Read the model definition and answer for the solid it produces. Units are mm, in the model's axes. A direction names the side the tool comes from. Coordinates: 2 decimals unless noted, no trailing zeros. Loops run counter-clockwise (first coordinate to the right, second up) from the corner with the lowest first, then second, coordinate; pieces in that order, holes last. Notation, with made-up numbers: M -0.75,75.25 L 18.25,75.25 A23 ccw 18.25,99.25 Z; hole C -33,81.25 d1. An arc over 180 degrees is marked long. One line per item, written item: value. Start each with the question number.
Autodesk Inventor part; units mm, degrees
ref_plane "YZ Plane" through (0, 0, 0) normal (1, 0, 0) x (0, 1, 0)
ref_plane "XZ Plane" through (0, 0, 0) normal (0, 1, 0) x (-1, 0, 0)
ref_plane "XY Plane" through (0, 0, 0) normal (0, 0, 1) x (1, 0, 0)
sketch "Sketch1" plane through (0, 0, 0) normal (0, 0, 1) x (1, 0, 0)
  line L0 (-20, 22.5) -> (20, 22.5)
  line L1 (20, 22.5) -> (20, -100)
  line L2 (20, -100) -> (-20, -100)
  line L3 (-20, -100) -> (-20, 22.5)
  circle A0 centre (0, 0) radius 4
  dimension "d0" = 122.5
  dimension "d1" = 40
  dimension "d2" = 20
  dimension "d3" = 22.5
  dimension "d4" = 8
extrude "Extrusion1" add sketch "Sketch1" along normal blind 5
sketch "Sketch2" plane through (0, 0, 5) normal (0, 0, 1) x (1, 0, 0)
  line L0 (20, 22.5) -> (-20, 22.5)
  line L1 (-20, -100) -> (20, -100)
  line L2 (-20, 22.5) -> (20, 22.5)
  line L3 (20, 22.5) -> (20, -100)
  line L4 (20, -100) -> (-20, -100)
  line L5 (-20, -100) -> (-20, 22.5)
  line L6 (-15, 17.5) -> (15, 17.5)
  line L7 (15, 17.5) -> (15, -95)
  line L8 (15, -95) -> (-15, -95)
  line L9 (-15, -95) -> (-15, 17.5)
  point P0 (0, 0)
  dimension "d7" = 5
  dimension "d8" = 5
  dimension "d9" = 5
  dimension "d10" = 5
extrude "Extrusion2" add sketch "Sketch2" along normal blind 35
sketch "Sketch3" plane through (-20, -100, 0) normal (0, -1, 0) x (1, 0, 0)
  circle A0 centre (20, 20) radius 4
  line L0 (40, 0) -> (40, 40)
  line L1 (0, 0) -> (40, 0)
  circle A1 centre (20, 20) radius 8.5
  line L2 (9.176, 20) -> (31.9076, 20)
  circle A2 centre (11.5, 20) radius 1.5
  circle A3 centre (28.5, 20) radius 1.5
  line L3 (0, 40) -> (40, 40)
  line L4 (20, 9.4564) -> (20, 30.2603)
  circle A4 centre (20, 28.5) radius 1.5
  circle A5 centre (20, 11.5) radius 1.5
  point P0 (20, 0)
  dimension "d13" = 20
  dimension "d14" = 20
  dimension "d15" = 8
  dimension "d16" = 17
  dimension "d17" = 3
  dimension "d18" = 3
  dimension "d19" = 20
  dimension "d20" = 20
  dimension "d21" = 3
  dimension "d22" = 3
extrude "Extrusion3" cut sketch "Sketch3" against normal blind 10 contours L2 L4 A0 | A0 L4 L2 | L4 L2 A0 | A0 L2 L4 | A4 A1 L4 | L4 A1 A4 | A5 A1 L4 | L4 A1 A5 | L4 A4 A1 | A1 A4 L4 | L4 A5 A1 | A1 A5 L4
sketch "Sketch4" plane through (-15, -95, 5) normal (0, 1, 0) x (1, 0, 0)
  line L0 (0, 0) -> (30, 0)
  line L1 (30, 0) -> (30, -35)
  line L2 (30, -35) -> (0, -35)
  line L3 (0, -35) -> (0, 0)
  circle A0 centre (15, -15) radius 4
  circle A1 centre (15, -15) radius 13
  circle A2 centre (15, -23.5) radius 1.5
  circle A3 centre (15, -23.5) radius 1.5
  circle A4 centre (15, -6.5) radius 1.5
  circle A5 centre (15, -6.5) radius 1.5
  point P0 (15, 5)
  dimension "d25" = 26
extrude "Extrusion4" add sketch "Sketch4" along normal blind 3 contours L0 L1 L2 L3 | A1
sketch "Sketch5" plane through (-15, -92, 5) normal (0, 1, 0) x (1, 0, 0)
  circle A0 centre (15, -15) radius 4
  circle A1 centre (15, -15) radius 13
  point P0 (15, 5)
  dimension "d28" = 26
extrude "Extrusion5" cut sketch "Sketch5" against normal blind 4
fillet "Fillet1" radius 2 5 edges at (-20, 22.5, 20) (20, 22.5, 20) (20, -100, 20) (-20, -100, 20) (20, -38.75, 0)
sketch "Sketch6" plane through (0, 0, 5) normal (0, 0, 1) x (1, 0, 0)
  line L0 (-15, -92) -> (-15, 17.5)
  line L1 (15, 17.5) -> (15, -92)
  line L2 (-15, 17.5) -> (15, 17.5)
  line L3 (15, 17.5) -> (15, -17.5)
  line L4 (15, -17.5) -> (-15, -17.5)
  line L5 (-15, -17.5) -> (-15, 17.5)
  circle A0 centre (0, 0) radius 4
  point P0 (-15, -17.5)
  dimension "d32" = 35
extrude "Extrusion6" add sketch "Sketch6" along normal blind 20
sketch "Sketch7" plane through (0, 0, 0) normal (0, 0, -1) x (-1, 0, 0)
  circle A0 centre (0, 0) radius 9.5
  dimension "d35" = 19
extrude "Extrusion7" cut sketch "Sketch7" against normal blind 12.5
sketch "Sketch8" plane through (0, 0, 0) normal (0, 0, -1) x (-1, 0, 0)
  circle A0 centre (0, 0) radius 4
  circle A1 centre (0, 0) radius 11.5
  dimension "d38" = 23
extrude "Extrusion8" cut sketch "Sketch8" against normal blind 6.5
sketch "Sketch9" plane through (0, 0, 25) normal (0, 0, 1) x (1, 0, 0)
  circle A0 centre (0, 0) radius 4
extrude "Extrusion9" add sketch "Sketch9" against normal blind 12.5
sketch "Sketch10" plane through (0, 0, 12.5) normal (0, 0, -1) x (-1, 0, 0)
  circle A0 centre (0, 0) radius 6.2
  line L0 (0, 6.2) -> (0, 0)
  line L1 (0, 0) -> (6.261, -3.6148)
  line L2 (0, 0) -> (-6.878, -3.971)
  circle A1 centre (0, 6.2) radius 1.45
  circle A2 centre (5.3694, -3.1) radius 1.45
  circle A3 centre (-5.3694, -3.1) radius 1.45
  dimension "d43" = 12.4
  dimension "d44" = 120
  dimension "d45" = 120
  dimension "d46" = 2.9
  dimension "d47" = 2.9
  dimension "d48" = 2.9
extrude "Extrusion10" cut sketch "Sketch10" against normal blind 12.5 contours A1 L0 A0 | A0 A1 | A2 A0 | A0 L1 A2 | L0 A1 A0 | A0 A2 L1 | A3 L2 A0 | A0 L2 A3 | A3 A0 L2 | A3 L2 A0
sketch "Sketch11" plane through (0, 0, 25) normal (0, 0, 1) x (1, 0, 0)
  circle A0 centre (5.3694, -3.1) radius 1.45
  circle A1 centre (5.3694, -3.1) radius 4
  circle A2 centre (-5.3694, -3.1) radius 1.45
  circle A3 centre (-5.3694, -3.1) radius 4
  circle A4 centre (0, 6.2) radius 1.45
  circle A5 centre (0, 6.2) radius 4
  point P0 (0, 0)
  dimension "d51" = 8
  dimension "d52" = 8
  dimension "d53" = 8
extrude "Extrusion11" cut sketch "Sketch11" against normal blind 7
properties part number "Link5_v2"
1) Section A-A (y = 6.2) is taken. Determine the outline of the cut face in (x, z), then the cut area to 3 significant figures.
2) Section D-D (y = -28) is taken. Determine the outline of the cut face in (x, z), then the cut area to 3 significant figures.
3) Consider line 1 along X through (y, z) = (-59, 21); line 2 along X through (y, z) = (-97.6, 28.5); line 3 along Z through (x, y) = (0, -98). Determine where each line is inside the solid, lowest interval first.
4) Section B-B (x = 0) is taken. Count the separate pieces of the cut face and the enclosed holes in it, then the cut area to 3 significant figures.
5) Section C-C (z = 28.5) is taken. Determine the outline of the cut face in (x, y), then the cut area to 3 significant figures.
6) For a pull along Y with two mould halves and no side action, classify faces 1 (the face through (0, 17.5, 32)), 2 (the face through (-0.521, -98.028, 23.966)) as released by +Y, released by -Y, zero draft, split by the parting line, or undercut.
7) A tool of negligible diameter and unlimited length cuts with its end or side. For faces 3 (the face through (3, -96, 17)), 4 (the face through (4, 9, 6.5)), 5 (the face through (-1, -38, 0)), 6 (the face through (0, -98, 10)), 7 (the face through (-1.554, -1.899, 21.549)), from which of +Z, -Z, +X, -X, +Y, -Y can it reach the whole face along a straight path? Write none if from no direction.
8) Flat-ended cylindrical pins translate along their axes: pin 1 (3.5 mm diameter, centred on x = -5.37, y = -3.1, fed in from -Z); pin 2 (4 mm diameter, centred on x = 6, y = -2, fed in from +Z); pin 3 (15 mm diameter, centred on x = 0, y = 0, fed in from +Z). Find the tip coordinate at first contact, or state that the pin passes through.
Results found:
1. outline: M -20,0 L -9.69,0 L -9.69,6.5 L -7.2,6.5 L -7.2,12.5 L -1.45,12.5 L -1.45,18 L -4,18 L -4,25 L -15,25 L -15,40 L -20,40 Z; M 1.45,12.5 L 7.2,12.5 L 7.2,6.5 L 9.69,6.5 L 9.69,0 L 18,0 A2 ccw 20,2 L 20,40 L 15,40 L 15,25 L 4,25 L 4,18 L 1.45,18 Z
1. area: 865 mm²
2. outline: M -20,0 L 18,0 A2 ccw 20,2 L 20,40 L 15,40 L 15,5 L -15,5 L -15,40 L -20,40 Z
2. area: 549 mm²
3. line 1: x = -20 to -15, 15 to 20
3. line 2: x = -20 to -1.5, 1.5 to 20
3. line 3: z = 0 to 10, 13 to 16, 24 to 27, 30 to 40
4. separate pieces: 5
4. enclosed holes: 0
4. area: 1,270 mm²
5. outline: M -20,-98 A2 ccw -18,-100 L -1.5,-100 L -1.5,-96 L -9.84,-96 L -9.84,-92 L -15,-92 L -15,17.5 L 15,17.5 L 15,-92 L 9.84,-92 L 9.84,-96 L 1.5,-96 L 1.5,-100 L 18,-100 A2 ccw 20,-98 L 20,20.5 A2 ccw 18,22.5 L -18,22.5 A2 ccw -20,20.5 Z
5. area: 1,520 mm²
6. face 1: undercut
6. face 2: zero draft
7. face 3: none
7. face 4: -Z
7. face 5: -Z, +X, -X, +Y, -Y
7. face 6: -Y
7. face 7: +Z
8. pin 1: stops at z = 12.5
8. pin 2: stops at z = 18
8. pin 3: stops at z = 25
